Check sheet for the modelled part. Datum: model origin and axes. Units: mm. A direction names the side the tool comes from. Round coordinates to 2 decimals unless told otherwise and drop trailing zeros. Order: outer loops, then holes, each group sorted by start corner. A loop starts at its lowest first (then second) coordinate and runs counter-clockwise, first axis right, second up. Notation, with made-up numbers: (-34, -8.75) -> (15, -8.75) arc R23 ccw to (15, 22.25) -> close; hole circle Ø10 at (15, 59.5). An arc over 180 degrees is marked (long way). Use CSV: the item, a comma, the result in double quotes.
```python
from build123d import *

# Parameters (mm, degrees)
SKETCH2_W                = 290
SKETCH2_H                = 30
SKETCH2_W_2              = 280
SKETCH2_H_2              = 25
BOSS_EXTRUDE1_DEPTH      = 23.28
SKETCH3_W                = 290
SKETCH3_H                = 30
BOSS_EXTRUDE2_DEPTH      = 3
SKETCH4_W                = 23.28
SKETCH4_H                = 25
CUT_EXTRUDE1_DEPTH       = 1
CUT_EXTRUDE1_DEPTH_BACK  = 291
BOSS_EXTRUDE3_DEPTH      = 2
BOSS_EXTRUDE3_DEPTH_BACK = 3
SKETCH6_R                = 10
CUT_EXTRUDE2_DEPTH       = 2
SKETCH7_R                = 1.275
CUT_EXTRUDE3_DEPTH       = 10
SKETCH8_W                = 290
SKETCH8_H                = 2.5
CUT_EXTRUDE4_DEPTH       = 12
BOSS_EXTRUDE4_DEPTH      = 15
ESQUISSE1_W              = 15
ESQUISSE1_H              = 2
BOSS_EXTRU_1_DEPTH       = 49
ESQUISSE2_R              = 1.275
BOSS_EXTRU_2_DEPTH       = 3
CONG_1_R                 = 4


with BuildPart() as part:
    # Sketch2 → Boss-Extrude1 (new body)
    with BuildSketch(Plane.XY.offset(1.715456747)):
        Rectangle(SKETCH2_W, SKETCH2_H)
        Rectangle(SKETCH2_W_2, SKETCH2_H_2, mode=Mode.SUBTRACT)
    extrude(amount=BOSS_EXTRUDE1_DEPTH)

    # Sketch3 → Boss-Extrude2 (add)
    with BuildSketch(Plane.XY.offset(24.995456747)):
        Rectangle(SKETCH3_W, SKETCH3_H)
    extrude(amount=BOSS_EXTRUDE2_DEPTH)

    # Sketch4 → Cut-Extrude1 (cut, two sides)
    with BuildSketch(Plane(origin=(145, 0, 0), x_dir=(0, 0, -1), z_dir=(1, 0, 0))) as cut_extrude1_sk:
        with Locations((-13.355456747, 0)):
            Rectangle(SKETCH4_W, SKETCH4_H)
    extrude(amount=CUT_EXTRUDE1_DEPTH, mode=Mode.SUBTRACT)
    extrude(cut_extrude1_sk.sketch, amount=-CUT_EXTRUDE1_DEPTH_BACK, mode=Mode.SUBTRACT)

    # Sketch5 → Boss-Extrude3 (add, two sides)
    with BuildSketch(Plane(origin=(-0.5, 0, 0), x_dir=(0, 0, -1), z_dir=(1, 0, 0))) as boss_extrude3_sk:
        with BuildLine():
            Line((-27.995456747, 0), (-27.995456747, 15))
            Line((-27.995456747, 15), (-72.715456747, 15))
            Line((-72.715456747, 15), (-80.215456747, 0))
            Line((-80.215456747, 0), (-80.215456747, -21.531619709))
            ThreePointArc((-80.215456747, -21.531619709), (-72.715456747, -45.15), (-65.215456747, -21.531619709))
            Line((-65.215456747, -21.531619709), (-65.215456747, 0))
            Line((-65.215456747, 0), (-27.995456747, 0))
        make_face()
    extrude(amount=BOSS_EXTRUDE3_DEPTH)
    extrude(boss_extrude3_sk.sketch, amount=-BOSS_EXTRUDE3_DEPTH_BACK)

    # Sketch6 → Cut-Extrude2 (cut)
    with BuildSketch(Plane(origin=(-3.5, 0, 0), x_dir=(0, 0, -1), z_dir=(1, 0, 0))):
        with Locations((-72.715456747, -32.15)):
            Circle(SKETCH6_R)
    extrude(amount=CUT_EXTRUDE2_DEPTH, mode=Mode.SUBTRACT)

    # Sketch7 → Cut-Extrude3 (cut)
    with BuildSketch(Plane.ZY.offset(3.5)):
        with Locations((72.715456747, -25.15)):
            Circle(SKETCH7_R)
        with Locations((79.715456747, -32.15)):
            Circle(SKETCH7_R)
        with Locations((72.715456747, -39.15)):
            Circle(SKETCH7_R)
        with Locations((65.715456747, -32.15)):
            Circle(SKETCH7_R)
    extrude(amount=-CUT_EXTRUDE3_DEPTH, mode=Mode.SUBTRACT)

    # Sketch8 → Cut-Extrude4 (cut)
    with BuildSketch(Plane(origin=(0, 0, 1.715456747), x_dir=(-1, 0, 0), z_dir=(0, 0, -1))):
        with Locations((0, -13.75)):
            Rectangle(SKETCH8_W, SKETCH8_H)
    extrude(amount=-CUT_EXTRUDE4_DEPTH, mode=Mode.SUBTRACT)

    # Sketch9 → Boss-Extrude4 (add)
    with BuildSketch(Plane(origin=(0, 15, 0), x_dir=(1, 0, 0), z_dir=(0, 1, 0))):
        Polygon((-3.5, -58.92224084), (-63.5, -27.995456747), (-41.673741056, -27.995456747), (-3.5, -47.671974209), align=None)
        Polygon((61.5, -27.995456747), (39.673741056, -27.995456747), (1.5, -47.671974209), (1.5, -58.92224084), align=None)
    extrude(amount=-BOSS_EXTRUDE4_DEPTH)

    # Esquisse1 → Boss.-Extru.1 (add)
    with BuildSketch(Plane.ZY.offset(3.5)):
        with Locations((72.715456747, -6.15)):
            Rectangle(ESQUISSE1_W, ESQUISSE1_H)
    extrude(amount=BOSS_EXTRU_1_DEPTH)

    # Esquisse2 → Boss.-Extru.2 (add)
    with BuildSketch(Plane.ZY.offset(52.5)):
        with BuildLine():
            Line((65.215456747, -21.531619709), (65.215456747, -25.535621722))
            ThreePointArc((65.215456747, -25.535621722), (72.715456747, -42.15), (80.215456747, -25.535621722))
            Line((80.215456747, -25.535621722), (80.215456747, -21.531619709))
            Line((80.215456747, -21.531619709), (80.215456747, -7.15))
            Line((80.215456747, -7.15), (80.215456747, -5.15))
            Line((80.215456747, -5.15), (65.215456747, -5.15))
            Line((65.215456747, -5.15), (65.215456747, -7.15))
            Line((65.215456747, -7.15), (65.215456747, -12.828367585))
            Line((65.215456747, -12.828367585), (65.215456747, -21.531619709))
        make_face()
        with Locations((72.715456747, -39.15)):
            Circle(ESQUISSE2_R, mode=Mode.SUBTRACT)
        with Locations((79.715456747, -32.15)):
            Circle(ESQUISSE2_R, mode=Mode.SUBTRACT)
        with Locations((72.715456747, -25.15)):
            Circle(ESQUISSE2_R, mode=Mode.SUBTRACT)
        with Locations((65.715456747, -32.15)):
            Circle(ESQUISSE2_R, mode=Mode.SUBTRACT)
    extrude(amount=BOSS_EXTRU_2_DEPTH)

    # Congé1
    cong_1_edges = [part.edges().sort_by_distance(p)[0] for p in [
        (-3.5, -7.15, 72.715456747),
        (-3.5, -5.15, 72.715456747),
        (-52.5, -7.15, 72.715456747),
        (-55.5, -5.15, 72.715456747),
    ]]
    fillet(cong_1_edges, radius=CONG_1_R)


solid = part.part
```
Q1. Mould release check, pull along Y, two halves, no side actions. Record for faces 4 (the face through (-53.979, -42.145, 72.394)), 5 (the face through (-28, -7.15, 73)), 6 (the face through (1.5, 8, 38)), 7 (the face through (-21, -7, 65.215)): pulls with the +Y half, pulls with the -Y half, needs draft (parallel to the pull), parting line crosses it, or undercut.
Result sheet:
face 4,"parting line crosses it"
face 5,"pulls with the -Y half"
face 6,"needs draft"
face 7,"undercut"
Q2. Sectioned sample at A-A, the plane x = -15.5. Enter the section's corners in (y, z).
Result sheet:
outline,"(-15, 13.72) -> (-12.5, 13.72) -> (-12.5, 25) -> (12.5, 25) -> (12.5, 1.72) -> (15, 1.72) -> (15, 28) -> (-15, 28) -> close; (-7.15, 65.22) -> (-5.15, 65.22) -> (-5.15, 80.22) -> (-7.15, 80.22) -> close; (0, 41.49) -> (15, 41.49) -> (15, 52.74) -> (0, 52.74) -> close"
Q3. Sectioned sample at C-C, the plane x = 65.5. Enter the section's corners in (y, z).
Result sheet:
outline,"(-15, 13.72) -> (-12.5, 13.72) -> (-12.5, 25) -> (12.5, 25) -> (12.5, 1.72) -> (15, 1.72) -> (15, 28) -> (-15, 28) -> close"
Q4. Sectioned sample at B-B, the plane z = 40. Enter the section's corners in (x, y).
Result sheet:
outline,"(-40.21, 0) -> (-18.38, 0) -> (-18.38, 15) -> (-40.21, 15) -> close; (-3.5, 0) -> (1.5, 0) -> (1.5, 15) -> (-3.5, 15) -> close; (16.38, 0) -> (38.21, 0) -> (38.21, 15) -> (16.38, 15) -> close"
Q5. Scan lines: L1, parallel to Z at x = -53, y = -32; L2, parallel to X at y = -37.5, z = 75.5; L3, parallel to X at y = 9.5, z = 35. Record each from-to range of solid material in increasing order.
Result sheet:
L1,"z = 62.72 to 64.45, 66.98 to 78.45, 80.98 to 82.71"
L2,"x = -55.5 to -52.5, -1.5 to 1.5"
L3,"x = -49.91 to -28.08, -3.5 to 1.5, 26.08 to 47.91"
Q6. Go/stop test with flat-tipped pins: pin 1 (22 mm diameter, centred on y = -23, z = 77.5, fed in from -X); pin 2 (4 mm diameter, centred on y = 1, z = 66, fed in from +X); pin 3 (18.5 mm diameter, centred on x = -33.5, z = 13.5, fed in from -Y). Record where each tip stops, or that it passes through.
Result sheet:
pin 1,"stops at x = -55.5"
pin 2,"stops at x = 1.5"
pin 3,"stops at y = -15"
Q7. Access from +Z, -Z, +X, -X, +Y, -Y to the whole of each face (thin tool, end or side, straight path). Record for faces 1 (the face through (-3.5, 8, 38)), 2 (the face through (2, 12.5, 14)), 3 (the face through (-3.5, -20, 73)).
Result sheet:
face 1,"+Y, -Y"
face 2,"-Z, +X, -X"
face 3,"+Z, -Y"
